from build123d import *

# Parameters (mm, degrees)
BASPROSKE_W         = 8
BASPROSKE_H         = 22
TOOTHCUT_DEPTH      = 33.124756808
TEETHCUTS_COUNT     = 20
TEETHCUTS_ANGLE     = 342
BORSKE_R            = 2
BORE_DEPTH          = 8
SKETCH1_R           = 14
CUT_EXTRUDE1_DEPTH  = 3
CUT_EXTRUDE2_DEPTH  = 32.859573128
BOSS_EXTRUDE1_DEPTH = 8
CUT_EXTRUDE3_DEPTH  = 66.194920127
CHAMFER1_SIZE       = 30


with BuildPart() as part:
    # BasProSke → Base-Revolve (revolve)
    with BuildSketch(Plane(origin=(0, 0, 0), x_dir=(1, 0, 0), z_dir=(0, 1, 0)), mode=Mode.PRIVATE) as base_revolve_sk:
        with Locations((4, 11)):
            Rectangle(BASPROSKE_W, BASPROSKE_H)
    revolve(base_revolve_sk.sketch.rotate(Axis((-10, 0, 0), (1, 0, 0)), 180), axis=Axis((-10, 0, 0), (1, 0, 0)))

    # TooCutSke → ToothCut (cut, through all)
    with BuildSketch(Plane(origin=(0, 0, 0), x_dir=(0, 0, -1), z_dir=(1, 0, 0))):
        with BuildLine():
            ThreePointArc((0.986171591, 17.471189616), (0, 17.499), (-0.986171591, 17.471189616))
            ThreePointArc((-0.986171591, 17.471189616), (-1.626916196, 19.798789858), (-2.932850173, 21.829260982))
            ThreePointArc((-2.932850173, 21.829260982), (0, 22.0254), (2.932850173, 21.829260982))
            ThreePointArc((2.932850173, 21.829260982), (1.626916196, 19.798789858), (0.986171591, 17.471189616))
        make_face()
    toothcut = extrude(amount=TOOTHCUT_DEPTH, mode=Mode.SUBTRACT)

    # TeethCuts: ToothCut ×20 about axis
    teethcuts_axis = Axis((-10, 0, 0), (1, 0, 0))
    for i in range(1, TEETHCUTS_COUNT):
        add(toothcut.rotate(teethcuts_axis, i * TEETHCUTS_ANGLE / (TEETHCUTS_COUNT - 1)), mode=Mode.SUBTRACT)

    # BorSke → Bore (cut, symmetric)
    with BuildSketch(Plane(origin=(0, 0, 0), x_dir=(0, 0, -1), z_dir=(1, 0, 0))):
        with Locations(Location((0, 0, 0), (0, 0, 180))):
            Circle(BORSKE_R)
    extrude(amount=BORE_DEPTH, both=True, mode=Mode.SUBTRACT)

    # Sketch1 → Cut-Extrude1 (cut)
    with BuildSketch(Plane(origin=(8, 0, 0), x_dir=(0, 0, -1), z_dir=(1, 0, 0))):
        Circle(SKETCH1_R)
    extrude(amount=-CUT_EXTRUDE1_DEPTH, mode=Mode.SUBTRACT)

    # Sketch2 → Cut-Extrude2 (cut, through all)
    with BuildSketch(Plane.ZY):
        Polygon((-21.592193025, -6.419793995), (20.580067201, 14.175220465), (12.820897061, 30.063616315), (-23.756341743, 14.175220465), (-26.106914947, 1.214231969), align=None)
    extrude(amount=-CUT_EXTRUDE2_DEPTH, mode=Mode.SUBTRACT)

    # Sketch3 → Boss-Extrude1 (add)
    with BuildSketch(Plane.ZY):
        Polygon((13.740882365, 10.835273546), (-49.159279282, -19.882305538), (-57.935730449, -1.910830782), (4.964431198, 28.806748303), align=None)
    extrude(amount=-BOSS_EXTRUDE1_DEPTH)

    # Sketch6 → Cut-Extrude3 (cut, through all)
    with BuildSketch(Plane(origin=(8, 0, 0), x_dir=(0, 0, -1), z_dir=(1, 0, 0))):
        Polygon((50.475746957, -17.186584325), (57.935730449, -1.910830782), (21.992780936, 15.642071552), align=None)
    extrude(amount=-CUT_EXTRUDE3_DEPTH, mode=Mode.SUBTRACT)

    # Chamfer1
    # the kernel refuses this chamfer: 30 mm, written as the material it takes off along each edge
    with BuildSketch(Plane(origin=(-77.150489639, 28.806748303, 4.964431198), x_dir=(0, -0.4139495743409253, -0.9102998131950631), z_dir=(1, 0, 0))) as chamfer1_piece_1_section:
        Polygon((CHAMFER1_SIZE * 0.999621916911, -CHAMFER1_SIZE * 0.0274958766106), (-CHAMFER1_SIZE * 0.0274958766106, -CHAMFER1_SIZE * 0.999621916911), (0, 0), align=None)
    chamfer1_piece_1 = extrude(amount=162.300979278, mode=Mode.PRIVATE)
    chamfer1_piece_1 = chamfer1_piece_1 - Plane(origin=(2.5, 0, 0), x_dir=(0, 0.632443978109164, 0.7746061028377297), z_dir=(-1, 0, 0)) * Cylinder(17.499, 445, mode=Mode.PRIVATE)
    chamfer1_piece_1 = split(chamfer1_piece_1, bisect_by=Plane(origin=(2.5, 5.973711679, 3.785897747), z_dir=(0, 0.898573737810962, -0.43882255834954154)), keep=Keep.TOP, mode=Mode.PRIVATE)
    add(chamfer1_piece_1, mode=Mode.SUBTRACT)


solid = part.part
Part model, mm, in its own coordinate system. A direction names the side the tool comes from. Coordinates: 2 decimals unless noted, no trailing zeros. Loops run counter-clockwise (first coordinate to the right, second up) from the corner with the lowest first, then second, coordinate; pieces in that order, holes last. Notation, with made-up numbers: M -25,5.5 L 32,5.5 A20 ccw 32,20.5 Z; hole C 80,17 d10. An arc over 180 degrees is marked long. Use a Markdown table: item, result. Add a question column.
Q1. Pin check, flat tips, straight feed: P1, Ø2, axis at x = 4, y = 2.5, coming from the -Z side; P2, Ø3, axis at x = 5, z = -20, coming from the -Y side; P3, Ø1, axis at x = 3.5, z = -42.5, coming from the -Y side. Stop position of each tip, or through.
Q2. Cut at B-B (z = 0). Write the cut outline in (x, y).
Q3. Cut at A-A (y = 0). Write the cut outline in (x, z).
Q4. Probe L1, parallel to Z at x = 2.75, y = -7; L2, parallel to Z at x = 4.75, y = -8.5; L3, parallel to Y at x = 6.25, z = -24.5. List the from-to ranges inside material, lowest first.
Q5. Cut at C-C (z = 8.5). Write the cut outline in (x, y).
Q6. Which spindle directions (+Z, -Z, +X, -X, +Y, -Y) get a long thin tool onto all of the face, cutting with end or side? Do faces 4 (the flat face through (5, -5, 3)), 5 (the cylindrical face through (3.94, -7.63, 18.29)), 6 (the cylindrical face through (3.94, -15.07, 12.97)), 7 (the cylindrical face through (3.944, -14.149, 10.297)). Say none if no direction does.
Q7. Mould opens along Z. For faces 1 (the flat face through (8, -2, -14)), 2 (the cylindrical face through (3.944, -1.607, 19.754)), 3 (the flat face through (6.48, 3.41, -1.46)) say: +Z half, -Z half, draft (parallel to the pull), parting line (faces both ways), or undercut.
Q8. Cut at D-D (z = -39). Write the cut outline in (x, y).
Worked out:
| question | item | result |
|---|---|---|
| 1 | P1 | stops at z = -34.26 |
| 1 | P2 | stops at y = -10.49 |
| 1 | P3 | stops at y = -16.87 |
| 2 | outline | M 0,-17.5 L 8,-17.5 L 8,-14 L 5,-14 L 5,-2 L 0,-2 Z; M 0,2 L 5,2 L 5,4.12 L 8,4.12 L 8,17.5 L 0,17.5 Z |
| 3 | outline | M 0,-35.56 L 8,-35.56 L 8,-8.45 L 5,-8.45 L 5,-2 L 0,-2 Z; M 0,2 L 5,2 L 5,14 L 8,14 L 8,17.5 L 0,17.5 Z |
| 4 | L1 | z = -41.64 to -22.78, -17.48 to 17.48 |
| 4 | L2 | z = -42.94 to -25.85, -19.13 to 19.13 |
| 4 | L3 | y = -7.84 to 12.75 |
| 5 | outline | M 0,-19.13 L 8,-19.13 L 8,-11.12 L 5,-11.12 L 5,8.28 L 8,8.28 L 8,15.3 L 0,15.3 Z |
| 6 | face 4 | +X |
| 6 | face 5 | +Z, +X, -X |
| 6 | face 6 | +X, -X, -Y |
| 6 | face 7 | +X, -X |
| 7 | face 1 | draft |
| 7 | face 2 | +Z half |
| 7 | face 3 | undercut |
| 8 | outline | M 0,-14.92 L 8,-14.92 L 8,-3.96 L 0,-3.96 Z |
